Build history of the part. All positions in model axes, mm. Give positions to 0.01 mm unless a question says otherwise; leave off trailing zeros. Write each loop counter-clockwise with the first axis right and the second up, starting at its lowest first coordinate (ties: lowest second). Pieces come first, ordered by that corner, then holes. Notation, with made-up numbers: (47, 81.25) -> (82, 81.25) arc R16 cw to (82, 102.25) -> close; hole circle Ø6 at (12, 86). An arc over 180 degrees is marked (long way). Put each result on its own line as item: value.
from build123d import *

# Parameters (mm, degrees)
BOSS_EXTRUDE1_DEPTH = 3
SKETCH2_W           = 16
SKETCH2_H           = 16
CUT_EXTRUDE1_DEPTH  = 3


with BuildPart() as part:
    # Sketch1 → Boss-Extrude1 (new body)
    with BuildSketch(Plane(origin=(0, 0, 0), x_dir=(1, 0, 0), z_dir=(0, 1, 0))):
        with BuildLine():
            Line((-8.396433729, 36.75), (8.396433729, 36.75))
            ThreePointArc((8.396433729, 36.75), (9.647519653, 36.310379445), (10.348602488, 35.184784011))
            Line((10.348602488, 35.184784011), (17.325497736, 3.858708099))
            ThreePointArc((17.325497736, 3.858708099), (0, -17.75), (-17.325497736, 3.858708099))
            Line((-17.325497736, 3.858708099), (-10.348602488, 35.184784011))
            ThreePointArc((-10.348602488, 35.184784011), (-9.647519653, 36.310379445), (-8.396433729, 36.75))
        make_face()
    extrude(amount=BOSS_EXTRUDE1_DEPTH)

    # Sketch2 → Cut-Extrude1 (cut)
    with BuildSketch(Plane(origin=(0, 3, 0), x_dir=(1, 0, 0), z_dir=(0, 1, 0))):
        Rectangle(SKETCH2_W, SKETCH2_H)
    extrude(amount=-CUT_EXTRUDE1_DEPTH, mode=Mode.SUBTRACT)


solid = part.part
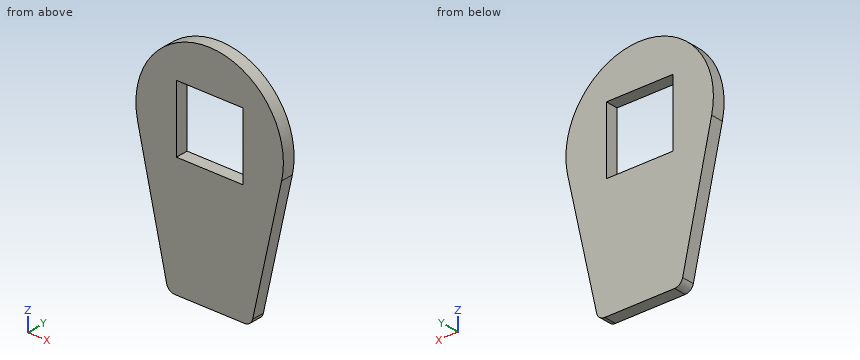
1) Slice it at D-D (z = -26). Write the cut outline in (x, y), plus the area to 3 significant figures.
Filled sheet:
outline: (-12.39, 0) -> (12.39, 0) -> (12.39, 3) -> (-12.39, 3) -> close
area: 74.4 mm2
2) Wall check: L1, parallel to X at y = 1.05, z = -5; L2, parallel to X at y = 0.95, z = 7.5; L3, parallel to Z at x = 3, y = 1. Give the ranges that are in metal, low to high.
Filled sheet:
L1: -17.07 to -8, 8 to 17.07
L2: -16.09 to -8, 8 to 16.09
L3: -36.75 to -8, 8 to 17.49
3) Slice it at B-B (y = 2.55). Write the cut outline in (x, z).
Filled sheet:
outline: (-17.33, -3.86) -> (-10.35, -35.18) arc R2 ccw to (-8.4, -36.75) -> (8.4, -36.75) arc R2 ccw to (10.35, -35.18) -> (17.33, -3.86) arc R17.75 ccw (long way) to start; hole (-8, -8) -> (8, -8) -> (8, 8) -> (-8, 8) -> close
4) Slice it at A-A (x = 0). Write the cut outline in (y, z), plus the area to 4 significant figures.
Filled sheet:
outline: (0, -36.75) -> (3, -36.75) -> (3, -8) -> (0, -8) -> close; (0, 8) -> (3, 8) -> (3, 17.75) -> (0, 17.75) -> close
area: 115.5 mm2
5) Pin check, flat tip, straight feed: pin 1 (1 mm diameter, centred on y = 1, z = -14.5, fed in from -X). Stop position of the tip, or through.
Filled sheet:
pin 1: x = -15.07
6) Slice it at C-C (z = 0). Write the cut outline in (x, y), plus the area to 3 significant figures.
Filled sheet:
outline: (-17.75, 0) -> (-8, 0) -> (-8, 3) -> (-17.75, 3) -> close; (8, 0) -> (17.75, 0) -> (17.75, 3) -> (8, 3) -> close
area: 58.5 mm2
